Geometry check sheet. Reference: drawing and pictorial views, mm from the part's lowest x, y, z. A direction names the side the tool comes from. Give positions to 0.01 mm unless a question says otherwise; leave off trailing zeros. Write each loop counter-clockwise with the first axis right and the second up, starting at its lowest first coordinate (ties: lowest second). Pieces come first, ordered by that corner, then holes. Notation, with made-up numbers: M 35,37.25 L 46,37.25 A37 cw 46,73.25 Z; hole C 15,67 d10. An arc over 180 degrees is marked long. One line per item, written item: value. Start each with the question number.
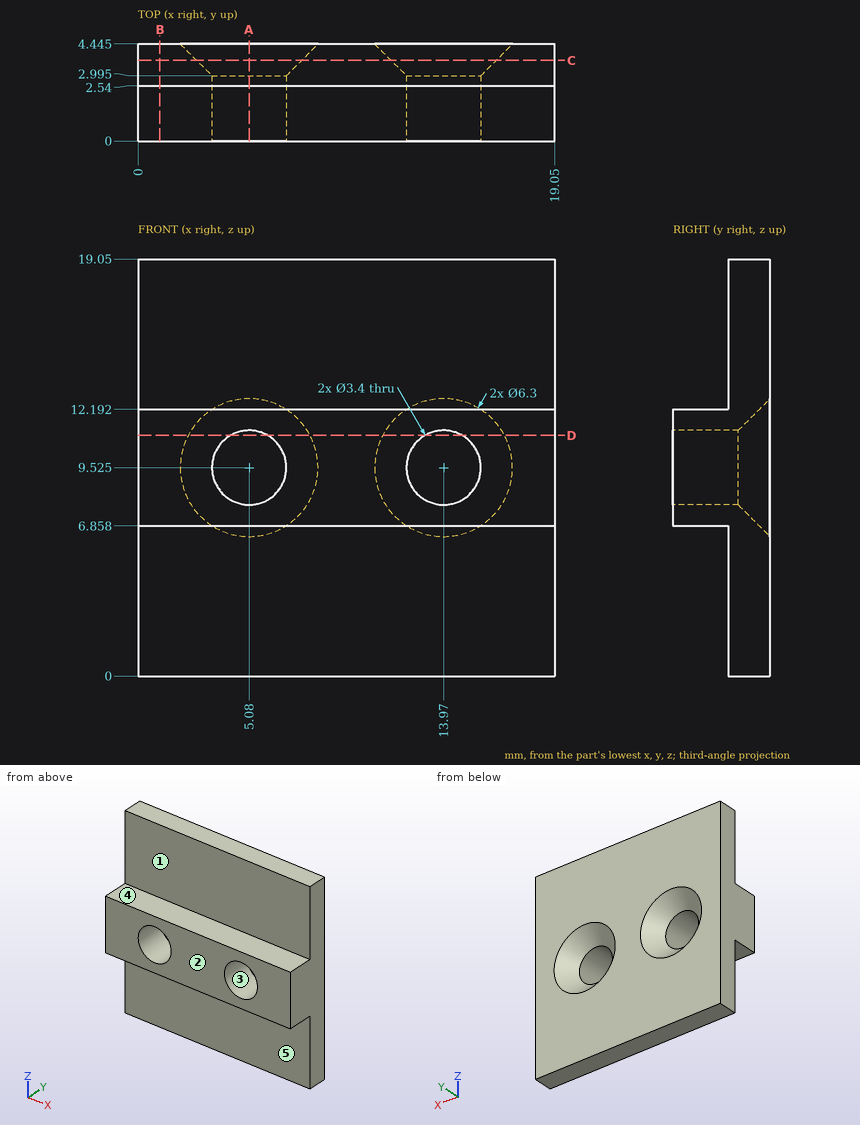
1) Cross-section at C-C (y = 3.7). Record the boundary of the cut face in (x, z) (3 decimals).
2) Tool access check on the marked faces 1 and 2. Record the directions out of +Z, -Z, +X, -X, +Y, -Y that give a thin tool (end or side, any length) a straight path to the whole face; none if there is none.
3) Cross-section at D-D (z = 11). State how many separate pieces and enclosed holes the cut face has, plus the area to 3 significant figures.
4) Cross-section at A-A (x = 5.08). Record the boundary of the cut face in (y, z) (3 decimals).
5) Draft check along Z on the marked faces 3, 4 and 5. Enter one of: released by +Z, released by -Z, zero draft, split by the parting line, or undercut.
6) Gauge pin test, flat ends, axial feed: pin 1 (3.5 mm diameter, centred on x = 10.5, z = 16.5, fed in from -Y); pin 2 (1.3 mm diameter, centred on x = 11, y = 1, fed in from -Z); pin 3 (2 mm diameter, centred on x = 6.5, y = 1.5, fed in from +Z). Record the tip position at first contact, or that the pin passes through.
7) Material ranges on L1, parallel to Z at x = 5.08, y = 2 (3 decimals); L2, parallel to Z at x = 8, y = 2.15; L3, parallel to Y at x = 9.5, z = 14.5 (3 decimals), recorded low to high. Write a range as from..to.
8) Cross-section at B-B (x = 1). Record the boundary of the cut face in (y, z) (3 decimals), plus the area to 3 significant figures.
Data:
1. outline: M 0,0 L 19.05,0 L 19.05,19.05 L 0,19.05 Z; hole C 5.08,9.525 d4.81; hole C 13.97,9.525 d4.81
2. face 1: +Z, +X, -X, -Y
2. face 2: +Z, -Z, +X, -X, -Y
3. separate pieces: 3
3. enclosed holes: 0
3. area: 63.6 mm2
4. outline: M 0,6.858 L 2.54,6.858 L 2.54,0 L 4.445,0 L 4.445,6.375 L 2.995,7.825 L 0,7.825 Z; M 0,11.225 L 2.995,11.225 L 4.445,12.675 L 4.445,19.05 L 2.54,19.05 L 2.54,12.192 L 0,12.192 Z
5. face 3: undercut
5. face 4: released by +Z
5. face 5: zero draft
6. pin 1: stops at y = 2.54
6. pin 2: stops at z = 6.86
6. pin 3: stops at z = 12.19
7. L1: z = 6.858..7.825, 11.225..12.192
7. L2: z = 6.86..12.19
7. L3: y = 2.54..4.445
8. outline: M 0,6.858 L 2.54,6.858 L 2.54,0 L 4.445,0 L 4.445,19.05 L 2.54,19.05 L 2.54,12.192 L 0,12.192 Z
8. area: 49.8 mm2
